Input: part model. Units: mm. Frame: model coordinates. A direction names the side the tool comes from. Coordinates: 2 decimals unless noted, no trailing zeros. Write each loop counter-clockwise with the first axis right and the second up, starting at its lowest first coordinate (ties: lowest second). Pieces come first, ordered by that corner, then holes.
from build123d import *

# Parameters (mm, degrees)
PCB_HOLDER_R             = 0.75
BOSS_EXTRUDE19_DEPTH     = 1
PCB_HOLDER_R_2           = 3
BOSS_EXTRUDE19_2_DEPTH   = 1
BOSS_EXTRUDE20_OUTLINE_R = 0.75
BOSS_EXTRUDE20_DEPTH     = 2
BOSS_EXTRUDE21_DEPTH     = 4
BOSS_EXTRUDE22_DEPTH     = 7
PCB_HOLDER_49_W          = 2.5
PCB_HOLDER_49_H          = 1
PCB_HOLDER_49_H_2        = 0.75
BOSS_EXTRUDE23_DEPTH     = 13.25
SKETCH10_W               = 2.5
SKETCH10_H               = 2
BOSS_EXTRUDE24_DEPTH     = 2
CUT_EXTRUDE9_DEPTH       = 20
CUT_EXTRUDE10_DEPTH      = 20
SKETCH9_W                = 9.5
SKETCH9_H                = 1.75
BOSS_EXTRUDE25_DEPTH     = 1.5
CUT_EXTRUDE11_DEPTH      = 10
CUT_EXTRUDE12_DEPTH      = 10
CUT_EXTRUDE13_DEPTH      = 10


# Read off the part's stored shape, not the designer's step: Boss-Extrude20
with BuildPart() as part:
    # PCB holder → Boss-Extrude19 (new body)
    with BuildSketch(Plane(origin=(0, 0, 0), x_dir=(1, 0, 0), z_dir=(0, 1, 0))):
        with BuildLine():
            Line((-10, -13.5), (-10, -10.5))
            Line((-10, -10.5), (-12, -10.5))
            ThreePointArc((-12, -10.5), (-13.5, -12), (-12, -13.5))
            Line((-12, -13.5), (-10, -13.5))
        make_face()
        with Locations(Location((-12, -12, 0), (0, 0, 270))):
            Circle(PCB_HOLDER_R, mode=Mode.SUBTRACT)
    extrude(amount=BOSS_EXTRUDE19_DEPTH)

    # Boss-Extrude20 outline → Boss-Extrude20 (add)
    with BuildSketch(Plane(origin=(0, 0, 0), x_dir=(1, 0, 0), z_dir=(0, 1, 0))):
        with BuildLine():
            Line((10, -14.5), (10, -13.5))
            Line((10, -13.5), (12, -13.5))
            ThreePointArc((12, -13.5), (13.5, -12), (12, -10.5))
            Line((12, -10.5), (10, -10.5))
            Line((10, -10.5), (10, 14.5))
            ThreePointArc((10, 14.5), (9.707106781, 15.207106781), (9, 15.5))
            Line((9, 15.5), (4.75, 15.5))
            Line((4.75, 15.5), (4.75, 17))
            Line((4.75, 17), (-4.75, 17))
            Line((-4.75, 17), (-4.75, 15.5))
            Line((-4.75, 15.5), (-9, 15.5))
            ThreePointArc((-9, 15.5), (-9.707106781, 15.207106781), (-10, 14.5))
            Line((-10, 14.5), (-10, -10.5))
            Line((-10, -10.5), (-12, -10.5))
            ThreePointArc((-12, -10.5), (-13.5, -12), (-12, -13.5))
            Line((-12, -13.5), (-10, -13.5))
            Line((-10, -13.5), (-10, -14.5))
            ThreePointArc((-10, -14.5), (-9.707106781, -15.207106781), (-9, -15.5))
            Line((-9, -15.5), (9, -15.5))
            ThreePointArc((9, -15.5), (9.707106781, -15.207106781), (10, -14.5))
        make_face()
        with Locations((12, -12)):
            Circle(BOSS_EXTRUDE20_OUTLINE_R, mode=Mode.SUBTRACT)
        with BuildLine():
            Line((-8.75, 14.75), (8.75, 14.75))
            ThreePointArc((8.75, 14.75), (9.103553391, 14.603553391), (9.25, 14.25))
            Line((9.25, 14.25), (9.25, -14.25))
            ThreePointArc((9.25, -14.25), (9.103553391, -14.603553391), (8.75, -14.75))
            Line((8.75, -14.75), (-8.75, -14.75))
            ThreePointArc((-8.75, -14.75), (-9.103553391, -14.603553391), (-9.25, -14.25))
            Line((-9.25, -14.25), (-9.25, 14.25))
            ThreePointArc((-9.25, 14.25), (-9.103553391, 14.603553391), (-8.75, 14.75))
        make_face(mode=Mode.SUBTRACT)
        with Locations((-12, -12)):
            Circle(BOSS_EXTRUDE20_OUTLINE_R, mode=Mode.SUBTRACT)
    extrude(amount=BOSS_EXTRUDE20_DEPTH)



with BuildPart() as body_2:
    # PCB holder → Boss-Extrude19 2 (new body)
    with BuildSketch(Plane(origin=(0, 0, 0), x_dir=(1, 0, 0), z_dir=(0, 1, 0))):
        with BuildLine():
            Line((8.75, 14.75), (-8.75, 14.75))
            ThreePointArc((-8.75, 14.75), (-9.103553391, 14.603553391), (-9.25, 14.25))
            Line((-9.25, 14.25), (-9.25, -14.25))
            ThreePointArc((-9.25, -14.25), (-9.103553391, -14.603553391), (-8.75, -14.75))
            Line((-8.75, -14.75), (7.5, -14.75))
            Line((7.5, -14.75), (7.5, -15.5))
            Line((7.5, -15.5), (9, -15.5))
            ThreePointArc((9, -15.5), (9.707106781, -15.207106781), (10, -14.5))
            Line((10, -14.5), (10, -13.5))
            Line((10, -13.5), (12, -13.5))
            ThreePointArc((12, -13.5), (13.5, -12), (12, -10.5))
            Line((12, -10.5), (10, -10.5))
            Line((10, -10.5), (10, 14.5))
            ThreePointArc((10, 14.5), (9.707106781, 15.207106781), (9, 15.5))
            Line((9, 15.5), (8.75, 15.5))
            Line((8.75, 15.5), (8.75, 14.75))
        make_face()
        with Locations(Location((0, -5, 0), (0, 0, 270))):
            Circle(PCB_HOLDER_R_2, mode=Mode.SUBTRACT)
        with Locations(Location((0, 5, 0), (0, 0, 270))):
            Circle(PCB_HOLDER_R_2, mode=Mode.SUBTRACT)
        with Locations(Location((12, -12, 0), (0, 0, 270))):
            Circle(PCB_HOLDER_R, mode=Mode.SUBTRACT)
    extrude(amount=BOSS_EXTRUDE19_2_DEPTH)

    # PCB holder<47> → Boss-Extrude21 (add)
    with BuildSketch(Plane(origin=(0, 0, 0), x_dir=(1, 0, 0), z_dir=(0, 1, 0))):
        with BuildLine():
            Line((9, 15.5), (-9, 15.5))
            ThreePointArc((-9, 15.5), (-9.707106781, 15.207106781), (-10, 14.5))
            Line((-10, 14.5), (-10, -14.5))
            ThreePointArc((-10, -14.5), (-9.707106781, -15.207106781), (-9, -15.5))
            Line((-9, -15.5), (9, -15.5))
            ThreePointArc((9, -15.5), (9.707106781, -15.207106781), (10, -14.5))
            Line((10, -14.5), (10, 14.5))
            ThreePointArc((10, 14.5), (9.707106781, 15.207106781), (9, 15.5))
        make_face()
        with BuildLine():
            Line((9.25, 14.25), (9.25, -14.25))
            ThreePointArc((9.25, -14.25), (9.103553391, -14.603553391), (8.75, -14.75))
            Line((8.75, -14.75), (-8.75, -14.75))
            ThreePointArc((-8.75, -14.75), (-9.103553391, -14.603553391), (-9.25, -14.25))
            Line((-9.25, -14.25), (-9.25, 14.25))
            ThreePointArc((-9.25, 14.25), (-9.103553391, 14.603553391), (-8.75, 14.75))
            Line((-8.75, 14.75), (8.75, 14.75))
            ThreePointArc((8.75, 14.75), (9.103553391, 14.603553391), (9.25, 14.25))
        make_face(mode=Mode.SUBTRACT)
    extrude(amount=BOSS_EXTRUDE21_DEPTH)

    # PCB holder<48> → Boss-Extrude22 (add)
    with BuildSketch(Plane(origin=(0, 0, 0), x_dir=(1, 0, 0), z_dir=(0, 1, 0))):
        Polygon((-4.75, 15.5), (-8.75, 15.5), (-8.75, 14.75), (8.75, 14.75), (8.75, 15.5), (4.75, 15.5), align=None)
    extrude(amount=BOSS_EXTRUDE22_DEPTH)


with BuildPart() as part_1:
    add(part.part)

    add(body_2.part)  # Boss-Extrude23 merges body 2
    # PCB holder<49> → Boss-Extrude23 (add)
    with BuildSketch(Plane(origin=(0, 0, 0), x_dir=(1, 0, 0), z_dir=(0, 1, 0))):
        with Locations((-6.25, -16)):
            Rectangle(PCB_HOLDER_49_W, PCB_HOLDER_49_H)
        with Locations((6.25, -16)):
            Rectangle(PCB_HOLDER_49_W, PCB_HOLDER_49_H)
        with Locations((-6.25, -15.125)):
            Rectangle(PCB_HOLDER_49_W, PCB_HOLDER_49_H_2)
        with Locations((6.25, -15.125)):
            Rectangle(PCB_HOLDER_49_W, PCB_HOLDER_49_H_2)
    extrude(amount=BOSS_EXTRUDE23_DEPTH)

    # Sketch10 → Boss-Extrude24 (add)
    with BuildSketch(Plane(origin=(0, 0, 14.75), x_dir=(-1, 0, 0), z_dir=(0, 0, -1))):
        with Locations((-6.25, 12.25)):
            Rectangle(SKETCH10_W, SKETCH10_H)
        with Locations((6.25, 12.25)):
            Rectangle(SKETCH10_W, SKETCH10_H)
    extrude(amount=BOSS_EXTRUDE24_DEPTH)

    # Sketch11 → Cut-Extrude9 (cut)
    with BuildSketch(Plane(origin=(7.5, 0, 0), x_dir=(0, 0, -1), z_dir=(1, 0, 0))):
        Polygon((-12.75, 11.25), (-14.625, 13.25), (-12.75, 13.25), align=None)
    extrude(amount=-CUT_EXTRUDE9_DEPTH, mode=Mode.SUBTRACT)

    # Sketch12 → Cut-Extrude10 (cut)
    with BuildSketch(Plane.ZY.offset(4.75)):
        Polygon((-15.5, 0), (-17, 2), (-17, 0), align=None)
    extrude(amount=-CUT_EXTRUDE10_DEPTH, mode=Mode.SUBTRACT)

    # Sketch9 → Boss-Extrude25 (add)
    with BuildSketch(Plane.XY.offset(-14.75)):
        with Locations((0, 6.125)):
            Rectangle(SKETCH9_W, SKETCH9_H)
    extrude(amount=BOSS_EXTRUDE25_DEPTH)

    # Sketch15 → Cut-Extrude11 (cut)
    with BuildSketch(Plane.ZY.offset(4.75)):
        Polygon((-14.75, 7), (-13.25, 5.25), (-13.25, 7), align=None)
    extrude(amount=-CUT_EXTRUDE11_DEPTH, mode=Mode.SUBTRACT)

    # Sketch16 → Cut-Extrude12 (cut)
    with BuildSketch(Plane.XY.offset(-14.75)):
        Polygon((8.75, 4), (4.75, 7), (8.75, 7), align=None)
    extrude(amount=-CUT_EXTRUDE12_DEPTH, mode=Mode.SUBTRACT)

    # Sketch17 → Cut-Extrude13 (cut)
    with BuildSketch(Plane.XY.offset(-14.75)):
        Polygon((-8.75, 4), (-4.75, 7), (-8.75, 7), align=None)
    extrude(amount=-CUT_EXTRUDE13_DEPTH, mode=Mode.SUBTRACT)


solid = part_1.part
Item 1: Pin query (flat end, axial travel): pin 1 Ø1 at (x, y) = (-11.5, 1) entering from -Z; pin 2 Ø3 at (y, z) = (2, -1) entering from +X; pin 3 Ø1.9 at (y, z) = (9.5, 15) entering from -X. Return the tip coordinate at first contact, or that it passes through.
Item 2: Section query C-C, the plane x = -6.75. Return loops of the section in (y, z) (3 decimals), then the cut area to 3 significant figures.
Item 3: Section query A-A, the plane y = 7.5. Return loops of the section in (x, z), then the cut area to 3 significant figures.
Item 4: Pull-direction query (Z, two-part tool) for faces 1 (the face through (-11.721, 0.986, 12.696)), 2 (the face through (6.268, 12.236, 13.674)), 3 (the face through (9.699, 1.972, 15.215)); classes: released by +Z, released by -Z, zero draft, split by the parting line, or undercut.
Item 5: Section query D-D, the plane x = -2.25. Return loops of the section in (y, z), then the cut area to 3 significant figures.
Item 6: Access query for faces 4 (the face through (5, 8, 16)), 5 (the face through (-6, 11.25, 14)), 6 (the face through (0, 3, -14.75)). Directions: +Z, -Z, +X, -X, +Y, -Y. A direction counts if a zero-diameter tool reaches every point of the face in a straight line with its end or side. Return the directions, or none.
Item 7: Section query B-B, the plane z = 5. Return loops of the section in (x, y).
Item 8: Material intervals for line 1 (X direction, y = 0.95, z = 12); line 2 (Z direction, x = 7, y = 5); line 3 (Y direction, x = 7, z = 11), sorted ascending.
The answers:
1. pin 1: stops at z = 10.5
1. pin 2: stops at x = 10
1. pin 3: stops at x = -7.5
2. outline: (0, -15.5) - (5.5, -15.5) - (5.5, -14.75) - (1, -14.75) - (1, 14.75) - (11.25, 14.75) - (11.25, 12.75) - (13.25, 14.625) - (13.25, 16.5) - (0, 16.5) - close
2. area: 58.9 mm2
3. outline: (-7.5, 14.75) - (-5, 14.75) - (-5, 16.5) - (-7.5, 16.5) - close; (5, 14.75) - (7.5, 14.75) - (7.5, 16.5) - (5, 16.5) - close
3. area: 8.75 mm2
4. face 1: undercut
4. face 2: released by -Z
4. face 3: released by +Z
5. outline: (0, -15.5) - (2, -17) - (2, -15.5) - (7, -15.5) - (7, -14.75) - (5.25, -13.25) - (5.25, -14.75) - (1, -14.75) - (1, -6.98) - (0, -6.98) - close; (0, -3.02) - (1, -3.02) - (1, 3.02) - (0, 3.02) - close; (0, 6.98) - (1, 6.98) - (1, 14.75) - (4, 14.75) - (4, 15.5) - (0, 15.5) - close
5. area: 32.6 mm2
6. face 4: +Z, +Y
6. face 5: -Z, +X, -X
6. face 6: none
7. outline: (-10, 0) - (-3, 0) - (-3, 1) - (-9.25, 1) - (-9.25, 4) - (-10, 4) - close; (3, 0) - (10, 0) - (10, 4) - (9.25, 4) - (9.25, 1) - (3, 1) - close
8. line 1: x = -13.5 to -12.75, -11.25 to 11.25, 12.75 to 13.5
8. line 2: z = -15.5 to -14.75, 14.75 to 16.5
8. line 3: y = 0 to 1
